CAD build for the part. Positions are in the model's coordinates, mm. A direction names the side the tool comes from. Give positions to 0.01 mm unless a question says otherwise; leave off trailing zeros. Loops run counter-clockwise (first coordinate to the right, second up) from the corner with the lowest first, then second, coordinate; pieces in that order, holes last.
```python
from build123d import *

# Parameters (mm, degrees)
SALIENTE_EXTRUIR1_DEPTH = 2
CROQUIS1_R              = 4
CORTAR_EXTRUIR1_DEPTH   = 2
CROQUIS2_R              = 1.5
CORTAR_EXTRUIR2_DEPTH   = 2
MATRIZC1_COUNT          = 4
CROQUIS4_R              = 4
CORTAR_EXTRUIR3_DEPTH   = 2
CROQUIS5_R              = 1.5
CORTAR_EXTRUIR4_DEPTH   = 2
MATRIZC2_COUNT          = 4


with BuildPart() as part:
    # Croquis3 → Saliente-Extruir1 (new body)
    with BuildSketch(Plane.XY):
        with BuildLine():
            Line((0, 15), (16.715728753, 15))
            ThreePointArc((16.715728753, 15), (18.629145914, 15.380602337), (20.251262658, 16.464466094))
            Line((20.251262658, 16.464466094), (39.393398282, 35.606601717))
            ThreePointArc((39.393398282, 35.606601717), (60.606601717, 35.606601717), (60.606601717, 14.393398282))
            Line((60.606601717, 14.393398282), (32.67766953, -13.535533906))
            ThreePointArc((32.67766953, -13.535533906), (31.055552786, -14.619397663), (29.142135624, -15))
            Line((29.142135624, -15), (0, -15))
            ThreePointArc((0, -15), (-15, 0), (0, 15))
        make_face()
    extrude(amount=SALIENTE_EXTRUIR1_DEPTH)

    # Croquis1 → Cortar-Extruir1 (cut)
    with BuildSketch(Plane.XY):
        Circle(CROQUIS1_R)
    extrude(amount=CORTAR_EXTRUIR1_DEPTH, mode=Mode.SUBTRACT)

    # Croquis2 → Cortar-Extruir2 (cut)
    with BuildSketch(Plane.XY):
        with Locations((0, 7.509798768)):
            Circle(CROQUIS2_R)
    cortar_extruir2 = extrude(amount=CORTAR_EXTRUIR2_DEPTH, mode=Mode.SUBTRACT)

    # MatrizC1: Cortar-Extruir2 ×4 about axis
    matrizc1_axis = Axis((0, 0, 0), (0, 0, 1))
    for i in range(1, MATRIZC1_COUNT):
        add(cortar_extruir2.rotate(matrizc1_axis, i * 360 / MATRIZC1_COUNT), mode=Mode.SUBTRACT)

    # Croquis4 → Cortar-Extruir3 (cut)
    with BuildSketch(Plane.XY.offset(2)):
        with Locations((50, 25)):
            Circle(CROQUIS4_R)
    extrude(amount=-CORTAR_EXTRUIR3_DEPTH, mode=Mode.SUBTRACT)

    # Croquis5 → Cortar-Extruir4 (cut)
    with BuildSketch(Plane.XY.offset(2)):
        with Locations((50, 32)):
            Circle(CROQUIS5_R)
    cortar_extruir4 = extrude(amount=-CORTAR_EXTRUIR4_DEPTH, mode=Mode.SUBTRACT)

    # MatrizC2: Cortar-Extruir4 ×4 about axis
    matrizc2_axis = Axis((50, 25, 0), (0, 0, 1))
    for i in range(1, MATRIZC2_COUNT):
        add(cortar_extruir4.rotate(matrizc2_axis, i * 360 / MATRIZC2_COUNT), mode=Mode.SUBTRACT)


solid = part.part
```
1. Saw through at A-A, the plane x = 50. List the corners of the cut face in (y, z).
Responses:
outline: (3.79, 0) - (16.5, 0) - (16.5, 2) - (3.79, 2) - close; (19.5, 0) - (21, 0) - (21, 2) - (19.5, 2) - close; (29, 0) - (30.5, 0) - (30.5, 2) - (29, 2) - close; (33.5, 0) - (40, 0) - (40, 2) - (33.5, 2) - close
2. Drop flat-ended pins along their axis: pin 1 (9 mm diameter, centred on x = 50, y = 25, fed in from +Z); pin 2 (1.8 mm diameter, centred on x = 0, y = 7.51, fed in from -Z); pin 3 (1 mm diameter, centred on x = 8, z = 0.5, fed in from +Y). Give the stop position or say it passes through.
Responses:
pin 1: stops at z = 2
pin 2: passes through
pin 3: stops at y = 15
3. Pull direction Y, two halves, no side cores. Call faces 3 (the face through (-15, 0, 1)), 4 (the face through (31.1, -14.6, 1)), 5 (the face through (44.464, 24.675, 1.014)): released by +Y, released by -Y, zero draft, split by the parting line, or undercut.
Responses:
face 3: split by the parting line
face 4: released by -Y
face 5: undercut
4. Tool access for faces 1 (the face through (-6.045, -0.325, 0.986)), 2 (the face through (8, 15, 1)): list every direction of +Z, -Z, +X, -X, +Y, -Y with a clear straight run to the whole face (end or side of a thin tool).
Responses:
face 1: +Z, -Z
face 2: +Z, -Z, -X, +Y
5. Saw through at D-D, the plane y = 32. List the corners of the cut face in (x, z), and give its area (3 significant figures).
Responses:
outline: (35.79, 0) - (48.5, 0) - (48.5, 2) - (35.79, 2) - close; (51.5, 0) - (63.27, 0) - (63.27, 2) - (51.5, 2) - close
area: 49.0 mm2
6. Saw through at B-B, the plane y = 0. List the corners of the cut face in (x, z).
Responses:
outline: (-15, 0) - (-9.01, 0) - (-9.01, 2) - (-15, 2) - close; (-6.01, 0) - (-4, 0) - (-4, 2) - (-6.01, 2) - close; (4, 0) - (6.01, 0) - (6.01, 2) - (4, 2) - close; (9.01, 0) - (46.21, 0) - (46.21, 2) - (9.01, 2) - close
7. Probe line 1 along Y through (x, z) = (0, 1.2); line 2 along Y through (x, z) = (50, 1.55); line 3 along X through (y, z) = (26, 1.3). List the from-to ranges inside material, lowest first.
Responses:
line 1: y = -15 to -9.01, -6.01 to -4, 4 to 6.01, 9.01 to 15
line 2: y = 3.79 to 16.5, 19.5 to 21, 29 to 30.5, 33.5 to 40
line 3: x = 29.79 to 41.88, 44.12 to 46.13, 53.87 to 55.88, 58.12 to 64.97
8. Saw through at C-C, the plane z = 1.65. Count the separate pieces of the cut face and the enclosed holes in it, and give its area (3 significant figures).
Responses:
separate pieces: 1
enclosed holes: 10
area: 2,360 mm2
